from build123d import *

# Parameters (mm, degrees)
SKETCH1_W           = 106.35
SKETCH1_H           = 121.35
SKETCH1_R           = 1.725
SKETCH1_R_2         = 6.35
BOSS_EXTRUDE1_DEPTH = 0.8
FILLET1_R           = 1


with BuildPart() as part:
    # Sketch1 → Boss-Extrude1 (new body)
    with BuildSketch(Plane.XY):
        with Locations((50, -57.5)):
            Rectangle(SKETCH1_W, SKETCH1_H)
        Circle(SKETCH1_R, mode=Mode.SUBTRACT)
        with Locations((100, 0)):
            Circle(SKETCH1_R, mode=Mode.SUBTRACT)
        with Locations((100, -115)):
            Circle(SKETCH1_R, mode=Mode.SUBTRACT)
        with Locations((0, -115)):
            Circle(SKETCH1_R, mode=Mode.SUBTRACT)
        with Locations((50, -57.5)):
            Circle(SKETCH1_R_2, mode=Mode.SUBTRACT)
    extrude(amount=BOSS_EXTRUDE1_DEPTH)

    # Fillet1
    fillet1_edges = [part.edges().sort_by_distance(p)[0] for p in [
        (-3.175, 3.175, 0.4),
        (103.175, 3.175, 0.4),
        (103.175, -118.175, 0.4),
        (-3.175, -118.175, 0.4),
    ]]
    fillet(fillet1_edges, radius=FILLET1_R)


solid = part.part
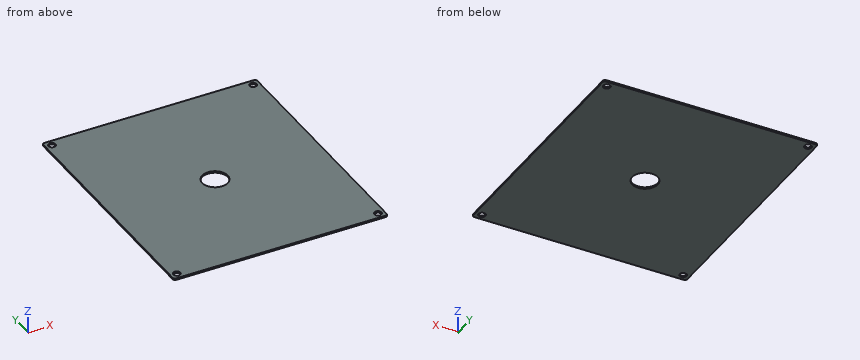
Model file for the job. Use its own axes, mm. Give positions to 0.01 mm unless a question says otherwise; leave off trailing zeros. Order: outer loops, then holes, each group sorted by start corner. A loop starts at its lowest first (then second) coordinate and runs counter-clockwise, first axis right, second up. Notation, with made-up numbers: M -22.5,-17.75 L -12.5,-17.75 A13 ccw -12.5,-1.75 Z; hole C 30.5,53 d10. An arc over 180 degrees is marked long. Write item = value, one per line.
Q1. Cut at D-D, the plane x = 51.5. List the corners of the cut face in (y, z) (3 decimals), then the cut area to 3 significant figures.
Derived:
outline = M -118.175,0 L -63.67,0 L -63.67,0.8 L -118.175,0.8 Z; M -51.33,0 L 3.175,0 L 3.175,0.8 L -51.33,0.8 Z
area = 87.2 mm2
Q2. Cut at B-B, the plane y = -115. List the corners of the cut face in (x, z) (3 decimals).
Derived:
outline = M -3.175,0 L -1.725,0 L -1.725,0.8 L -3.175,0.8 Z; M 1.725,0 L 98.275,0 L 98.275,0.8 L 1.725,0.8 Z; M 101.725,0 L 103.175,0 L 103.175,0.8 L 101.725,0.8 Z
Q3. Cut at A-A, the plane y = -57.5. List the corners of the cut face in (x, z) (3 decimals).
Derived:
outline = M -3.175,0 L 43.65,0 L 43.65,0.8 L -3.175,0.8 Z; M 56.35,0 L 103.175,0 L 103.175,0.8 L 56.35,0.8 Z
Q4. Drill centre lines: line 1 (Y direction, x = 0, z = 0.45) (3 decimals); line 2 (X direction, y = -115, z = 0.55) (3 decimals); line 3 (Y direction, x = 50, z = 0.65) (3 decimals). Where is each one in solid material? Low to high. Write a range as [from, to].
Derived:
line_1 = [-118.175, -116.725], [-113.275, -1.725], [1.725, 3.175]
line_2 = [-3.175, -1.725], [1.725, 98.275], [101.725, 103.175]
line_3 = [-118.175, -63.85], [-51.15, 3.175]
Q5. Cut at C-C, the plane x = 0. List the corners of the cut face in (y, z) (3 decimals).
Derived:
outline = M -118.175,0 L -116.725,0 L -116.725,0.8 L -118.175,0.8 Z; M -113.275,0 L -1.725,0 L -1.725,0.8 L -113.275,0.8 Z; M 1.725,0 L 3.175,0 L 3.175,0.8 L 1.725,0.8 Z
Q6. Flat gauge pin, fed straight in: pin 1 (2 mm diameter, centred on x = 100, y = 0, fed in from +Z). Where does the tip first touch, or does it go through?
Derived:
pin_1 = through
